from build123d import *

# Parameters (mm, degrees)
SKETCH1_W           = 100
SKETCH1_H           = 100
BOSS_EXTRUDE1_DEPTH = 100
SKETCH3_R           = 10
CUT_EXTRUDE1_DEPTH  = 10
SKETCH4_R           = 10
CUT_EXTRUDE2_DEPTH  = 10
FILLET5_R           = 5


with BuildPart() as part:
    # Sketch1 → Boss-Extrude1 (new body)
    with BuildSketch(Plane(origin=(0, 0, 0), x_dir=(1, 0, 0), z_dir=(0, 1, 0))):
        with Locations((50, 50)):
            Rectangle(SKETCH1_W, SKETCH1_H)
    extrude(amount=BOSS_EXTRUDE1_DEPTH)

    # Sketch3 → Cut-Extrude1 (cut)
    with BuildSketch(Plane(origin=(0, 0, -100), x_dir=(-1, 0, 0), z_dir=(0, 0, -1))):
        with Locations((-50, 50)):
            Circle(SKETCH3_R)
    extrude(amount=-CUT_EXTRUDE1_DEPTH, mode=Mode.SUBTRACT)

    # Sketch4 → Cut-Extrude2 (cut)
    with BuildSketch(Plane.XZ):
        with Locations(Location((21.715728753, -78.284271247, 0), (0, 0, 270))):
            Circle(SKETCH4_R)
        with Locations(Location((21.715728753, -21.715728753, 0), (0, 0, 270))):
            Circle(SKETCH4_R)
        with Locations(Location((78.284271247, -78.284271247, 0), (0, 0, 270))):
            Circle(SKETCH4_R)
        with Locations(Location((78.284271247, -21.715728753, 0), (0, 0, 270))):
            Circle(SKETCH4_R)
        with Locations(Location((50, -50, 0), (0, 0, 270))):
            Circle(SKETCH4_R)
    extrude(amount=-CUT_EXTRUDE2_DEPTH, mode=Mode.SUBTRACT)

    # Fillet5
    fillet5_edges = [part.edges().sort_by_distance(p)[0] for p in [
        (100, 100, -50),
        (50, 100, -100),
        (0, 100, -50),
        (50, 0, -100),
        (100, 0, -50),
        (50, 0, 0),
        (0, 0, -50),
        (0, 50, -100),
        (100, 50, -100),
        (100, 50, 0),
        (0, 50, 0),
        (50, 100, 0),
    ]]
    fillet(fillet5_edges, radius=FILLET5_R)


solid = part.part
Could you check a few things on this model? Use its own coordinates, in mm. A direction names the side the tool comes from. Coordinates: 2 decimals unless noted, no trailing zeros. Order: outer loops, then holes, each group sorted by start corner. A loop starts at its lowest first (then second) coordinate and runs counter-clockwise, first axis right, second up. Notation, with made-up numbers: (-6, -33.5) - (28, -33.5) arc R25 ccw to (28, -1.5) - close; hole circle Ø2 at (56, -6). An arc over 180 degrees is marked (long way). Answer in a Markdown table with one row per item. Add a question column.
(1) Will this pin go through, and if not, where does the flat tip stop? pin 1 (12 mm diameter, centred on x = 21.72, z = -78.28, fed in from -Y).
(2) On a 3-axis mill with a long thin cutter (end or side, diameter ignored), from which of +Z, -Z, +X, -X, +Y, -Y can I reach the whole of each face in a straight line? I mean faces 1 (the face through (1, 51, -98)), 2 (the face through (52.17, 40.24, -95.07)), 3 (the face through (22, 10, -78)). Say none if no direction works.
(3) If we section it at C-C, the plane x = 50: Please give me the cut outline in (y, z), then the cut area to 3 significant figures.
(4) If we mould it in two halves opening along Z, with no side actions, what happens to faces 4 (the face through (98, 1, -51)), 5 (the face through (40.24, 4.93, -47.83)), 6 (the face through (15.63, 4.93, -70.35)), 7 (the face through (51, 98, -99))? For each: released by +Z, released by -Z, zero draft, split by the parting line, or undercut.
(5) If we section it at A-A, the plane y = 50: Please give me the cut outline in (x, z).
(6) If we section it at D-D, the plane x = 18: Please give me the cut outline in (y, z), then the cut area to 3 significant figures.
(7) If we section it at B-B, the plane z = -50: Please give me the cut outline in (x, y), then the cut area to 3 significant figures.
(8) I need wall thicknesses on L1, parallel to Z at x = 77, y = 5.5; L2, parallel to Z at x = 71.5, y = 9.5; L3, parallel to Y at x = 50, z = -98. Which ranges of each line are inside material? Lowest first, please.
Results are:
| question | item | result |
|---|---|---|
| 1 | pin 1 | stops at y = 10 |
| 2 | face 1 | -Z, -X, +Y, -Y |
| 2 | face 2 | -Z |
| 2 | face 3 | -Y |
| 3 | outline | (0, -95) arc R5 ccw to (5, -100) - (40, -100) - (40, -90) - (60, -90) - (60, -100) - (95, -100) arc R5 ccw to (100, -95) - (100, -5) arc R5 ccw to (95, 0) - (5, 0) arc R5 ccw to (0, -5) - (0, -40) - (10, -40) - (10, -60) - (0, -60) - close |
| 3 | area | 9,580 mm2 |
| 4 | face 4 | zero draft |
| 4 | face 5 | undercut |
| 4 | face 6 | undercut |
| 4 | face 7 | released by -Z |
| 5 | outline | (0, -95) arc R5 ccw to (5, -100) - (40, -100) - (40, -90) - (60, -90) - (60, -100) - (95, -100) arc R5 ccw to (100, -95) - (100, -5) arc R5 ccw to (95, 0) - (5, 0) arc R5 ccw to (0, -5) - close |
| 6 | outline | (0, -95) arc R5 ccw to (5, -100) - (95, -100) arc R5 ccw to (100, -95) - (100, -5) arc R5 ccw to (95, 0) - (5, 0) arc R5 ccw to (0, -5) - (0, -12.43) - (10, -12.43) - (10, -31) - (0, -31) - (0, -69) - (10, -69) - (10, -87.57) - (0, -87.57) - close |
| 6 | area | 9,610 mm2 |
| 7 | outline | (0, 5) arc R5 ccw to (5, 0) - (40, 0) - (40, 10) - (60, 10) - (60, 0) - (95, 0) arc R5 ccw to (100, 5) - (100, 95) arc R5 ccw to (95, 100) - (5, 100) arc R5 ccw to (0, 95) - close |
| 7 | area | 9,780 mm2 |
| 8 | L1 | z = -100 to -88.2, -68.37 to -31.63, -11.8 to 0 |
| 8 | L2 | z = -100 to -85.63, -70.94 to -29.06, -14.37 to 0 |
| 8 | L3 | y = 1 to 40, 60 to 99 |
